Can you work these out from the model? Positions are in its coordinate system, mm. A direction names the side the tool comes from. Coordinates: 2 decimals unless noted, no trailing zeros. Order: outer loops, then holes, each group sorted by start corner. A loop starts at its lowest first (then second) coordinate and runs counter-clockwise, first axis right, second up.
```python
from build123d import *

# Parameters (mm, degrees)
BASE_FLANGE1_DEPTH  = 6
HEM2_DEPTH          = 160
SKETCH12_W          = 160
SKETCH12_H          = 6
BOSS_EXTRUDE2_DEPTH = 65.18
SKETCH13_W          = 37
SKETCH13_H          = 6
BOSS_EXTRUDE3_DEPTH = 48.91
SKETCH14_W          = 80
SKETCH14_H          = 6
BOSS_EXTRUDE4_DEPTH = 3
BOSS_EXTRUDE5_DEPTH = 80


# Read off the part's stored shape, not the designer's step: Hem2
# Sheet-metal steps are written as plain solids
with BuildPart() as part:
    # Sketch1 → Base-Flange1 (new body)
    with BuildSketch(Plane.XY):
        with BuildLine():
            Line((0, 0), (160, 0))
            Line((160, 0), (160, -144.47))
            ThreePointArc((160, -144.47), (159.87085305, -146.071955078), (159.486747986, -147.632532633))
            Line((159.486747986, -147.632532633), (122.276747986, -259.252532633))
            ThreePointArc((122.276747986, -259.252532633), (118.636993829, -264.202500426), (112.79, -266.09))
            Line((112.79, -266.09), (85, -266.09))
            Line((85, -266.09), (85, -251.09))
            ThreePointArc((85, -251.09), (80, -246.09), (75, -251.09))
            Line((75, -251.09), (75, -266.09))
            Line((75, -266.09), (47.21, -266.09))
            ThreePointArc((47.21, -266.09), (41.363006171, -264.202500426), (37.723252014, -259.252532633))
            Line((37.723252014, -259.252532633), (0.513252014, -147.632532633))
            ThreePointArc((0.513252014, -147.632532633), (0.12914695, -146.071955078), (0, -144.47))
            Line((0, -144.47), (0, 0))
        make_face()
        with BuildLine():
            Line((87.5, -173.59), (87.5, -223.59))
            ThreePointArc((87.5, -223.59), (80, -231.09), (72.5, -223.59))
            Line((72.5, -223.59), (72.5, -173.59))
            ThreePointArc((72.5, -173.59), (80, -166.09), (87.5, -173.59))
        make_face(mode=Mode.SUBTRACT)
    extrude(amount=-BASE_FLANGE1_DEPTH)

    # Hem2 outline → Hem2 (add)
    with BuildSketch(Plane.YZ):
        with BuildLine():
            Line((11.91, -17.91), (17.91, -17.91))
            ThreePointArc((17.91, -17.91), (12.664282451, -5.245717549), (0, 0))
            Line((0, 0), (0, -6))
            ThreePointArc((0, -6), (8.421641764, -9.488358236), (11.91, -17.91))
        make_face()
    extrude(amount=HEM2_DEPTH)

    # Sketch12 → Boss-Extrude2 (add)
    with BuildSketch(Plane(origin=(0, 0, -17.91), x_dir=(-1, 0, 0), z_dir=(0, 0, -1))):
        with Locations((-80, 14.91)):
            Rectangle(SKETCH12_W, SKETCH12_H)
    extrude(amount=BOSS_EXTRUDE2_DEPTH)

    # Sketch13 → Boss-Extrude3 (add)
    with BuildSketch(Plane(origin=(0, 0, -83.09), x_dir=(-1, 0, 0), z_dir=(0, 0, -1))):
        with Locations((-141.5, 14.91)):
            Rectangle(SKETCH13_W, SKETCH13_H)
        with Locations((-18.5, 14.91)):
            Rectangle(SKETCH13_W, SKETCH13_H)
    extrude(amount=BOSS_EXTRUDE3_DEPTH)

    # Sketch14 → Boss-Extrude4 (add)
    with BuildSketch(Plane(origin=(0, 0, -83.09), x_dir=(-1, 0, 0), z_dir=(0, 0, -1))):
        with Locations((-80, 14.91)):
            Rectangle(SKETCH14_W, SKETCH14_H)
    extrude(amount=BOSS_EXTRUDE4_DEPTH)

    # Sketch19 → Boss-Extrude5 (add)
    with BuildSketch(Plane(origin=(120, 0, 0), x_dir=(0, 0, -1), z_dir=(1, 0, 0))):
        with BuildLine():
            Line((98, 29.82), (98, 97.91))
            Line((98, 97.91), (104, 97.91))
            Line((104, 97.91), (104, 29.82))
            ThreePointArc((104, 29.82), (98.754282451, 17.155717549), (86.09, 11.91))
            Line((86.09, 11.91), (86.09, 17.91))
            ThreePointArc((86.09, 17.91), (94.511641764, 21.398358236), (98, 29.82))
        make_face()
    extrude(amount=-BOSS_EXTRUDE5_DEPTH)


solid = part.part
```
1. I'm going to push flat-ended pins straight in: pin 1 (3 mm diameter, centred on y = -260.5, z = -3, fed in from -X); pin 2 (16.5 mm diameter, centred on y = 37.5, z = -94, fed in from -X); pin 3 (3 mm diameter, centred on y = -255.5, z = -4.5, fed in from +X). Where does each tip first touch, or does it pass through?
Completed:
pin 1: stops at x = 37.64
pin 2: stops at x = 40
pin 3: stops at x = 124.03
2. On a 3-axis mill with a long thin cutter (end or side, diameter ignored), from which of +Z, -Z, +X, -X, +Y, -Y can I reach the whole of each face in a straight line? I mean faces 4 (the cylindrical face through (80.56, 17.296, -98.893)), 5 (the cylindrical face through (79.84, -166.09, -2.96)), 6 (the flat face through (81, 63, -98)). Say none if no direction works.
Completed:
face 4: -Z, -Y
face 5: +Z, -Z
face 6: +Z, +X, -X, +Y
3. Imagine slicing it at B-B on x = 139. Please give me the cut outline in (y, z), then the cut area to 3 significant figures.
Completed:
outline: (-209.09, -6) - (0, -6) arc R11.91 cw to (11.91, -17.91) - (11.91, -132) - (17.91, -132) - (17.91, -17.91) arc R17.91 ccw to (0, 0) - (-209.09, 0) - close
area: 2,080 mm2
4. Imagine slicing it at C-C on z = -21.5. Please give me the cut outline in (x, y), then the cut area to 3 significant figures.
Completed:
outline: (0, 11.91) - (160, 11.91) - (160, 17.91) - (0, 17.91) - close
area: 960 mm2
5. Please list where these lines run through material, in increasing order: probe 1 along Y at (x, z) = (104.5, -67); probe 2 along Z at (x, y) = (42, -245); probe 3 along Z at (x, y) = (67, 35).
Completed:
probe 1: y = 11.91 to 17.91
probe 2: z = -6 to 0
probe 3: z = -104 to -98
6. Imagine slicing it at D-D on y = -117. Please give me the cut outline in (x, z).
Completed:
outline: (0, -6) - (160, -6) - (160, 0) - (0, 0) - close
7. Thinking about a two-plate mould opening in X: for faces 1 (the flat face through (40, 46, -98.3)), 2 (the flat face through (141.142, -202.661, -2.958)), 3 (the cylindrical face through (78.88, 8.33, -9.4)), which applies, pulls with the +X half, pulls with the -X half, needs draft (parallel to the pull), parting line crosses it, or undercut?
Completed:
face 1: undercut
face 2: pulls with the +X half
face 3: needs draft
8. Imagine slicing it at A-A on x = 80. Please give me the cut outline in (y, z), then the cut area to 3 significant figures.
Completed:
outline: (-246.09, -6) - (-231.09, -6) - (-231.09, 0) - (-246.09, 0) - close; (-166.09, -6) - (0, -6) arc R11.91 cw to (11.91, -17.91) - (11.91, -86.09) arc R17.91 ccw to (29.82, -104) - (97.91, -104) - (97.91, -98) - (29.82, -98) arc R11.91 cw to (17.91, -86.09) - (17.91, -17.91) arc R17.91 ccw to (0, 0) - (-166.09, 0) - close
area: 2,190 mm2
